Verification items for the finished model (mm, model axes). Face numbers are marked on the shaded views. A direction names the side the tool comes from. Coordinates: 2 decimals unless noted, no trailing zeros. Write each loop counter-clockwise with the first axis right and the second up, starting at its lowest first coordinate (ties: lowest second). Pieces come first, ordered by that corner, then holes. Notation, with made-up numbers: (83.5, -12.5) -> (99.5, -12.5) arc R9 cw to (99.5, -2.5) -> close; hole circle Ø6 at (29.5, 45). An arc over 180 degrees is marked (long way). Answer in a Markdown table with one row per item.
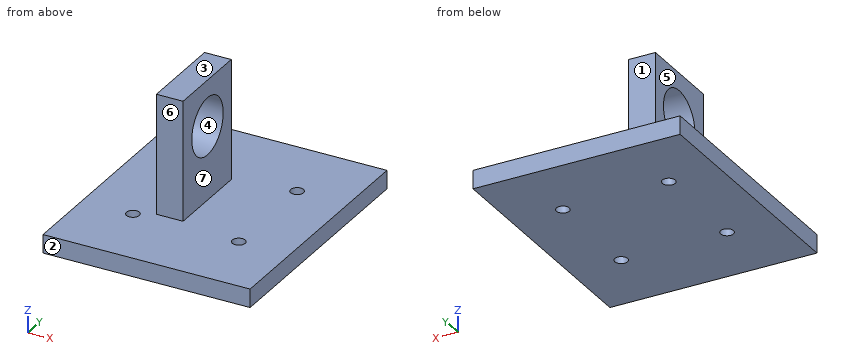
```python
from build123d import *

# Parameters (mm, degrees)
F0_W     = 45
F0_H     = 54
F0_R     = 1.4
F0_W_2   = 5.8
F0_H_2   = 19
F1_DEPTH = 4
F2_DEPTH = 30
F3_R     = 6.2
F4_DEPTH = 25


with BuildPart() as f1:
    # F0 (on Top) → F1 (new body)
    with BuildSketch(Plane.XY):
        with Locations((22.5, 27)):
            Rectangle(F0_W, F0_H)
        with Locations((11, 15.5)):
            Circle(F0_R, mode=Mode.SUBTRACT)
        with Locations((34, 15.5)):
            Circle(F0_R, mode=Mode.SUBTRACT)
        with Locations((11, 38.5)):
            Circle(F0_R, mode=Mode.SUBTRACT)
        with Locations((17.9, 27)):
            Rectangle(F0_W_2, F0_H_2, mode=Mode.SUBTRACT)
        with Locations((34, 38.5)):
            Circle(F0_R, mode=Mode.SUBTRACT)
    extrude(amount=F1_DEPTH)

    # F0 (on Top) → F2 (join)
    with BuildSketch(Plane.XY):
        with Locations((17.9, 27)):
            Rectangle(F0_W_2, F0_H_2)
    extrude(amount=F2_DEPTH)

    # F3 (on Right) → F4 (cut)
    with BuildSketch(Plane.YZ):
        with Locations((27.128499, 20)):
            Circle(F3_R)
    extrude(amount=F4_DEPTH, mode=Mode.SUBTRACT)


solid = f1.part
```
1. Section check C-C, the plane x = 34. Record the boundary of the cut face in (y, z).
Geometry says:
| item | result |
|---|---|
| outline | (0, 0) -> (14.1, 0) -> (14.1, 4) -> (0, 4) -> close; (16.9, 0) -> (37.1, 0) -> (37.1, 4) -> (16.9, 4) -> close; (39.9, 0) -> (54, 0) -> (54, 4) -> (39.9, 4) -> close |
2. Thickness scan on line 1 (Y direction, x = 11, z = 1.85); line 2 (Y direction, x = 16.9, z = 20); line 3 (Z direction, x = 43, y = 14.5). Record the ranges inside material, lowest first. Write a range as from..to.
Geometry says:
| item | result |
|---|---|
| line 1 | 0..14.1, 16.9..37.1, 39.9..54 |
| line 2 | 17.5..20.93, 33.33..36.5 |
| line 3 | 0..4 |
3. Section check B-B, the plane y = 38.5. Record the boundary of the cut face in (x, z).
Geometry says:
| item | result |
|---|---|
| outline | (0, 0) -> (9.6, 0) -> (9.6, 4) -> (0, 4) -> close; (12.4, 0) -> (32.6, 0) -> (32.6, 4) -> (12.4, 4) -> close; (35.4, 0) -> (45, 0) -> (45, 4) -> (35.4, 4) -> close |
4. Tool access check on the marked faces 5, 6 and 7. Record the directions out of +Z, -Z, +X, -X, +Y, -Y that give a thin tool (end or side, any length) a straight path to the whole face; none if there is none.
Geometry says:
| item | result |
|---|---|
| face 5 | +Z, -X, +Y, -Y |
| face 6 | +Z, +X, -X, -Y |
| face 7 | +Z, +X, +Y, -Y |
5. Mould release check, pull along Y, two halves, no side actions. Record for the marked faces 1, 2, 3 and 4: released by +Y, released by -Y, zero draft, split by the parting line, or undercut.
Geometry says:
| item | result |
|---|---|
| face 1 | released by +Y |
| face 2 | released by -Y |
| face 3 | zero draft |
| face 4 | undercut |
6. Section check A-A, the plane z = 20. Record the boundary of the cut face in (x, y).
Geometry says:
| item | result |
|---|---|
| outline | (15, 17.5) -> (20.8, 17.5) -> (20.8, 20.93) -> (15, 20.93) -> close; (15, 33.33) -> (20.8, 33.33) -> (20.8, 36.5) -> (15, 36.5) -> close |
7. Depth check by flat-ended pin: P1, Ø6.5, axis at x = 19, z = 22.5, coming from the -Y side; P2, Ø12, axis at y = 26, z = 15, coming from the +X side; P3, Ø3, axis at x = 17, z = 14, coming from the +Y side. Enter the tip coordinate at first touch or a pass-through.
Geometry says:
| item | result |
|---|---|
| P1 | y = 17.5 |
| P2 | x = 20.8 |
| P3 | y = 36.5 |
8. Section check D-D, the plane y = 20. Record the boundary of the cut face in (x, z), plus the area to 3 significant figures.
Geometry says:
| item | result |
|---|---|
| outline | (0, 0) -> (45, 0) -> (45, 4) -> (20.8, 4) -> (20.8, 30) -> (15, 30) -> (15, 4) -> (0, 4) -> close |
| area | 331 mm^2 |
